Design review of the part built by this model. Coordinates are the model's own, in mm. Face numbers are marked on the shaded views. Give positions to 0.01 mm unless a question says otherwise; leave off trailing zeros. Write each loop counter-clockwise with the first axis right and the second up, starting at its lowest first coordinate (ties: lowest second). Pieces come first, ordered by that corner, then holes. Notation, with made-up numbers: M 18,36 L 37,36 A17 cw 37,55 Z; hole C 38.25,19 d4. An arc over 180 degrees is marked long. Answer in a Markdown table with one row per item.
```python
from build123d import *

# Parameters (mm, degrees)
SKETCH_1_R      = 6
SKETCH_1_R_2    = 2.5
EXTRUDE_1_DEPTH = 3.2
CHAMFER_1_SIZE  = 2.7
FILLET_1_R      = 0.1


with BuildPart() as part:
    # 草图1 → 凸台-拉伸1 (new body)
    with BuildSketch(Plane(origin=(0, 0, 0), x_dir=(1, 0, 0), z_dir=(0, 1, 0))):
        with Locations(Location((0, 0, 0), (0, 0, 270))):
            Circle(SKETCH_1_R)
        with Locations(Location((0, 0, 0), (0, 0, 270))):
            Circle(SKETCH_1_R_2, mode=Mode.SUBTRACT)
    extrude(amount=EXTRUDE_1_DEPTH)

    # 倒角1
    chamfer_1_edges = [part.edges().sort_by_distance(p)[0] for p in [
        (0, 3.2, -2.5),
    ]]
    chamfer(chamfer_1_edges, length=CHAMFER_1_SIZE)

    # 圆角1
    fillet_1_edges = [part.edges().sort_by_distance(p)[0] for p in [
        (0, 3.2, -5.2),
        (0, 3.2, -6),
        (0, 0.5, -2.5),
    ]]
    fillet(fillet_1_edges, radius=FILLET_1_R)


solid = part.part
```
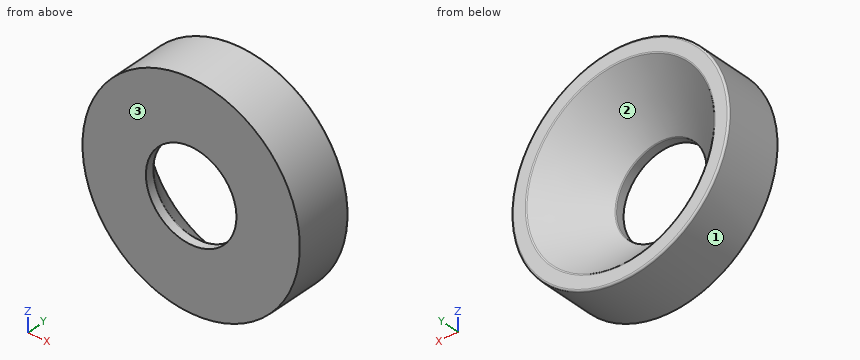
1) To check wall thickness, follow probe 1 along X at (y, z) = (0.3, 0); probe 2 along X at (y, z) = (1.65, -1.75); probe 3 along Z at (x, y) = (1.5, 1.15). State the ranges of each line that lie inside material, in increasing order. Write a range as [from, to].
Geometry says:
| item | result |
|---|---|
| probe 1 | [-6, -2.5], [2.5, 6] |
| probe 2 | [-5.74, -3.2], [3.2, 5.74] |
| probe 3 | [-5.81, -2.77], [2.77, 5.81] |
2) Add section B-B (y = 1.1). Write out the cut boundary in (x, z), and give its area (3 significant figures).
Geometry says:
| item | result |
|---|---|
| outline | C 0,0 d12; hole C 0,0 d6.2 |
| area | 82.9 mm^2 |
3) The part is to be moulded in two halves that separate along Z. For the marked faces 1, 2 and 3, say which applies: released by +Z, released by -Z, zero draft, split by the parting line, or undercut.
Geometry says:
| item | result |
|---|---|
| face 1 | split by the parting line |
| face 2 | undercut |
| face 3 | zero draft |
4) Insertion check: P1, Ø1, axis at x = 4.5, z = 1, coming from the +Y side; P2, Ø6.5, axis at x = 0, z = 0, coming from the +Y side. Each pin has a flat end and moves straight along its axis. Give the tip position at first contact, or say it passes through.
Geometry says:
| item | result |
|---|---|
| P1 | y = 3.11 |
| P2 | y = 1.25 |
5) Add section A-A (y = 2.2). Write out the cut boundary in (x, z).
Geometry says:
| item | result |
|---|---|
| outline | C 0,0 d12; hole C 0,0 d8.4 |
